from build123d import *

# Parameters (mm, degrees)
F1_DEPTH     = 25
F2_T1_DEPTH  = 30
F2_T3_DEPTH  = 30
F2_T5_DEPTH  = 30
F2_T7_DEPTH  = 30
F2_T9_DEPTH  = 30
F2_T11_DEPTH = 30
F2_T13_DEPTH = 30
F2_T15_DEPTH = 30
F2_T17_DEPTH = 30
F2_T19_DEPTH = 30
F2_T21_DEPTH = 30
F2_T23_DEPTH = 60.3553390593
F2_T25_DEPTH = 75


# Not quite as in the source:
# - a fillet or chamfer that OpenCascade refuses, or shapes differently, is made with other operations: its cross-section is extruded or revolved along the edge and cut away or added


with BuildPart() as f1:
    # F0 (on Top) → F1 (new body, symmetric)
    with BuildSketch(Plane.XY):
        Polygon((-96.1758106947, -16.0049479455), (-96.1758106947, -21.0049479455), (103.8241893053, -21.0049479455), (103.8241893053, -16.0049479455), (98.8241893053, -16.0049479455), (84.3241893053, -16.0049479455), (79.3241893053, -16.0049479455), (64.8241893053, -16.0049479455), (59.8241893053, -16.0049479455), (45.3241893053, -16.0049479455), (40.3241893053, -16.0049479455), (25.8241893053, -16.0049479455), (20.8241893053, -16.0049479455), (6.3241893053, -16.0049479455), (1.3241893053, -16.0049479455), (-13.1758106947, -16.0049479455), (-18.1758106947, -16.0049479455), (-32.6758106947, -16.0049479455), (-37.6758106947, -16.0049479455), (-52.1758106947, -16.0049479455), (-57.1758106947, -16.0049479455), (-71.6758106947, -16.0049479455), (-76.6758106947, -16.0049479455), (-91.1758106947, -16.0049479455), align=None)
        Polygon((-51.1758106947, 28.9950520545), (-96.1758106947, -16.0049479455), (-91.1758106947, -16.0049479455), (-46.1758106947, 28.9950520545), align=None)
        Polygon((98.8241893053, -16.0049479455), (103.8241893053, -16.0049479455), (148.8241893053, 28.9950520545), (143.8241893053, 28.9950520545), align=None)
        Polygon((-31.6758106947, 28.9950520545), (-76.6758106947, -16.0049479455), (-71.6758106947, -16.0049479455), (-26.6758106947, 28.9950520545), align=None)
        Polygon((79.3241893053, -16.0049479455), (84.3241893053, -16.0049479455), (129.3241893053, 28.9950520545), (124.3241893053, 28.9950520545), align=None)
        Polygon((-12.1758106947, 28.9950520545), (-57.1758106947, -16.0049479455), (-52.1758106947, -16.0049479455), (-7.1758106947, 28.9950520545), align=None)
        Polygon((59.8241893053, -16.0049479455), (64.8241893053, -16.0049479455), (109.8241893053, 28.9950520545), (104.8241893053, 28.9950520545), align=None)
        Polygon((7.3241893053, 28.9950520545), (-37.6758106947, -16.0049479455), (-32.6758106947, -16.0049479455), (12.3241893053, 28.9950520545), align=None)
        Polygon((40.3241893053, -16.0049479455), (45.3241893053, -16.0049479455), (90.3241893053, 28.9950520545), (85.3241893053, 28.9950520545), align=None)
        Polygon((26.8241893053, 28.9950520545), (-18.1758106947, -16.0049479455), (-13.1758106947, -16.0049479455), (31.8241893053, 28.9950520545), align=None)
        Polygon((20.8241893053, -16.0049479455), (25.8241893053, -16.0049479455), (70.8241893053, 28.9950520545), (65.8241893053, 28.9950520545), align=None)
        Polygon((46.3241893053, 28.9950520545), (1.3241893053, -16.0049479455), (6.3241893053, -16.0049479455), (51.3241893053, 28.9950520545), align=None)
    extrude(amount=F1_DEPTH, both=True)

    # F2: fillet of radius 5 on 25 edges, made by hand

    # F2_s2 → F2_t1 (cut)
    with BuildSketch(Plane.YZ.offset(-63.6758106947)):
        with BuildLine():
            ThreePointArc((28.9950520545, 20), (27.5305859605, 23.5355339059), (23.9950520545, 25))
            Line((23.9950520545, 25), (28.9950520545, 25))
            Line((28.9950520545, 25), (28.9950520545, 20))
        make_face()
        with BuildLine():
            ThreePointArc((28.9950520545, -20), (27.5305859605, -23.5355339059), (23.9950520545, -25))
            Line((23.9950520545, -25), (28.9950520545, -25))
            Line((28.9950520545, -25), (28.9950520545, -20))
        make_face()
    extrude(amount=F2_T1_DEPTH, mode=Mode.SUBTRACT)

    # F2_s4 → F2_t3 (cut)
    with BuildSketch(Plane.YZ.offset(-44.1758106947)):
        with BuildLine():
            ThreePointArc((28.9950520545, 20), (27.5305859605, 23.5355339059), (23.9950520545, 25))
            Line((23.9950520545, 25), (28.9950520545, 25))
            Line((28.9950520545, 25), (28.9950520545, 20))
        make_face()
        with BuildLine():
            ThreePointArc((28.9950520545, -20), (27.5305859605, -23.5355339059), (23.9950520545, -25))
            Line((23.9950520545, -25), (28.9950520545, -25))
            Line((28.9950520545, -25), (28.9950520545, -20))
        make_face()
    extrude(amount=F2_T3_DEPTH, mode=Mode.SUBTRACT)

    # F2_s6 → F2_t5 (cut)
    with BuildSketch(Plane.YZ.offset(-24.6758106947)):
        with BuildLine():
            ThreePointArc((28.9950520545, 20), (27.5305859604, 23.5355339059), (23.9950520545, 25))
            Line((23.9950520545, 25), (28.9950520545, 25))
            Line((28.9950520545, 25), (28.9950520545, 20))
        make_face()
        with BuildLine():
            ThreePointArc((28.9950520545, -20), (27.5305859604, -23.5355339059), (23.9950520545, -25))
            Line((23.9950520545, -25), (28.9950520545, -25))
            Line((28.9950520545, -25), (28.9950520545, -20))
        make_face()
    extrude(amount=F2_T5_DEPTH, mode=Mode.SUBTRACT)

    # F2_s8 → F2_t7 (cut)
    with BuildSketch(Plane.YZ.offset(-5.1758106947)):
        with BuildLine():
            ThreePointArc((28.9950520545, 20), (27.5305859604, 23.5355339059), (23.9950520545, 25))
            Line((23.9950520545, 25), (28.9950520545, 25))
            Line((28.9950520545, 25), (28.9950520545, 20))
        make_face()
        with BuildLine():
            ThreePointArc((28.9950520545, -20), (27.5305859604, -23.5355339059), (23.9950520545, -25))
            Line((23.9950520545, -25), (28.9950520545, -25))
            Line((28.9950520545, -25), (28.9950520545, -20))
        make_face()
    extrude(amount=F2_T7_DEPTH, mode=Mode.SUBTRACT)

    # F2_s10 → F2_t9 (cut)
    with BuildSketch(Plane.YZ.offset(14.3241893053)):
        with BuildLine():
            ThreePointArc((28.9950520545, 20), (27.5305859605, 23.5355339059), (23.9950520545, 25))
            Line((23.9950520545, 25), (28.9950520545, 25))
            Line((28.9950520545, 25), (28.9950520545, 20))
        make_face()
        with BuildLine():
            ThreePointArc((28.9950520545, -20), (27.5305859605, -23.5355339059), (23.9950520545, -25))
            Line((23.9950520545, -25), (28.9950520545, -25))
            Line((28.9950520545, -25), (28.9950520545, -20))
        make_face()
    extrude(amount=F2_T9_DEPTH, mode=Mode.SUBTRACT)

    # F2_s12 → F2_t11 (cut)
    with BuildSketch(Plane.YZ.offset(33.8241893053)):
        with BuildLine():
            ThreePointArc((28.9950520545, 20), (27.5305859605, 23.5355339059), (23.9950520545, 25))
            Line((23.9950520545, 25), (28.9950520545, 25))
            Line((28.9950520545, 25), (28.9950520545, 20))
        make_face()
        with BuildLine():
            ThreePointArc((28.9950520545, -20), (27.5305859605, -23.5355339059), (23.9950520545, -25))
            Line((23.9950520545, -25), (28.9950520545, -25))
            Line((28.9950520545, -25), (28.9950520545, -20))
        make_face()
    extrude(amount=F2_T11_DEPTH, mode=Mode.SUBTRACT)

    # F2_s14 → F2_t13 (cut)
    with BuildSketch(Plane.YZ.offset(53.3241893053)):
        with BuildLine():
            ThreePointArc((28.9950520545, 20), (27.5305859605, 23.5355339059), (23.9950520545, 25))
            Line((23.9950520545, 25), (28.9950520545, 25))
            Line((28.9950520545, 25), (28.9950520545, 20))
        make_face()
        with BuildLine():
            ThreePointArc((28.9950520545, -20), (27.5305859605, -23.5355339059), (23.9950520545, -25))
            Line((23.9950520545, -25), (28.9950520545, -25))
            Line((28.9950520545, -25), (28.9950520545, -20))
        make_face()
    extrude(amount=F2_T13_DEPTH, mode=Mode.SUBTRACT)

    # F2_s16 → F2_t15 (cut)
    with BuildSketch(Plane.YZ.offset(72.8241893053)):
        with BuildLine():
            ThreePointArc((28.9950520545, 20), (27.5305859605, 23.5355339059), (23.9950520545, 25))
            Line((23.9950520545, 25), (28.9950520545, 25))
            Line((28.9950520545, 25), (28.9950520545, 20))
        make_face()
        with BuildLine():
            ThreePointArc((28.9950520545, -20), (27.5305859605, -23.5355339059), (23.9950520545, -25))
            Line((23.9950520545, -25), (28.9950520545, -25))
            Line((28.9950520545, -25), (28.9950520545, -20))
        make_face()
    extrude(amount=F2_T15_DEPTH, mode=Mode.SUBTRACT)

    # F2_s18 → F2_t17 (cut)
    with BuildSketch(Plane.YZ.offset(92.3241893053)):
        with BuildLine():
            ThreePointArc((28.9950520545, 20), (27.5305859605, 23.5355339059), (23.9950520545, 25))
            Line((23.9950520545, 25), (28.9950520545, 25))
            Line((28.9950520545, 25), (28.9950520545, 20))
        make_face()
        with BuildLine():
            ThreePointArc((28.9950520545, -20), (27.5305859605, -23.5355339059), (23.9950520545, -25))
            Line((23.9950520545, -25), (28.9950520545, -25))
            Line((28.9950520545, -25), (28.9950520545, -20))
        make_face()
    extrude(amount=F2_T17_DEPTH, mode=Mode.SUBTRACT)

    # F2_s20 → F2_t19 (cut)
    with BuildSketch(Plane.YZ.offset(111.8241893053)):
        with BuildLine():
            ThreePointArc((28.9950520545, 20), (27.5305859605, 23.5355339059), (23.9950520545, 25))
            Line((23.9950520545, 25), (28.9950520545, 25))
            Line((28.9950520545, 25), (28.9950520545, 20))
        make_face()
        with BuildLine():
            ThreePointArc((28.9950520545, -20), (27.5305859605, -23.5355339059), (23.9950520545, -25))
            Line((23.9950520545, -25), (28.9950520545, -25))
            Line((28.9950520545, -25), (28.9950520545, -20))
        make_face()
    extrude(amount=F2_T19_DEPTH, mode=Mode.SUBTRACT)

    # F2_s22 → F2_t21 (cut)
    with BuildSketch(Plane.YZ.offset(131.3241893053)):
        with BuildLine():
            ThreePointArc((28.9950520545, 20), (27.5305859605, 23.5355339059), (23.9950520545, 25))
            Line((23.9950520545, 25), (28.9950520545, 25))
            Line((28.9950520545, 25), (28.9950520545, 20))
        make_face()
        with BuildLine():
            ThreePointArc((28.9950520545, -20), (27.5305859605, -23.5355339059), (23.9950520545, -25))
            Line((23.9950520545, -25), (28.9950520545, -25))
            Line((28.9950520545, -25), (28.9950520545, -20))
        make_face()
    extrude(amount=F2_T21_DEPTH, mode=Mode.SUBTRACT)

    # F2_s24 → F2_t23 (cut)
    with BuildSketch(Plane.XY.offset(-30.1776695297)):
        with BuildLine():
            ThreePointArc((-96.1758106947, -18.0760157573), (-95.7952083573, -16.1625985955), (-94.7113446006, -14.5404818514))
            Line((-94.7113446006, -14.5404818514), (-96.1758106947, -16.0049479455))
            Line((-96.1758106947, -16.0049479455), (-96.1758106947, -18.0760157573))
        make_face()
    extrude(amount=F2_T23_DEPTH, mode=Mode.SUBTRACT)

    # F2_s26 → F2_t25 (cut)
    with BuildSketch(Plane.XY.offset(-37.5)):
        with BuildLine():
            ThreePointArc((-96.1758106947, -16.0049479455), (-94.7113446006, -19.5404818514), (-91.1758106947, -21.0049479455))
            Line((-91.1758106947, -21.0049479455), (-96.1758106947, -21.0049479455))
            Line((-96.1758106947, -21.0049479455), (-96.1758106947, -16.0049479455))
        make_face()
        with BuildLine():
            ThreePointArc((103.8241893053, -16.0049479455), (102.3597232112, -19.5404818514), (98.8241893053, -21.0049479455))
            Line((98.8241893053, -21.0049479455), (103.8241893053, -21.0049479455))
            Line((103.8241893053, -21.0049479455), (103.8241893053, -16.0049479455))
        make_face()
    extrude(amount=F2_T25_DEPTH, mode=Mode.SUBTRACT)


solid = f1.part
Here's how the part is built. I have some questions about the finished solid (model axes, mm). A direction names the side the tool comes from. Give positions to 0.01 mm unless a question says otherwise; leave off trailing zeros. Order: outer loops, then holes, each group sorted by start corner. A loop starts at its lowest first (then second) coordinate and runs counter-clockwise, first axis right, second up. Notation, with made-up numbers: (2, -3.5) -> (11, -3.5) arc R15 cw to (11, 25.5) -> close; hole circle Ø1 at (77, 65). An arc over 180 degrees is marked (long way). Use a Markdown table: item, result. Add a question column.
Item 1: I need wall thicknesses on line 1 (Y direction, x = -19, z = 15); line 2 (Y direction, x = 96.5, z = -8.5); line 3 (Y direction, x = 9, z = -22). Which ranges of each line are inside material? Lowest first, please.
Item 2: Imagine slicing it at A-A on x = 57. Please give me the cut outline in (y, z).
Item 3: Will these pins go through, and if not, where does the flat tip stop? pin 1 (4 mm diameter, centred on x = -48.5, y = -14.5, fed in from +Z); pin 2 (4.5 mm diameter, centred on x = 94.5, z = -5, fed in from +Y); pin 3 (1 mm diameter, centred on x = -21.5, z = -3.5, fed in from +Y); pin 4 (11.5 mm diameter, centred on x = -83.5, z = -11, fed in from +Y).
Item 4: For faces 5 (the face through (-30.635, 27.569, 23.496)), 6 (the face through (48.01, 6.18, 0.35)), which set-ups out of +Z, -Z, +X, -X, +Y, -Y let a thin tool reach every point of the face, with its end or its side?
Item 5: Imagine slicing it at B-B on y = -7. Give the number of separate pieces and of enclosed holes in the cut face, plus the area to 3 significant figures.
Item 6: If we mould it in two halves opening along Y, with no side actions, what happens to faces 1 (the face through (-94.36, -19.86, -0.35)), 2 (the face through (-68.99, 6.18, 0.35)), 3 (the face through (-14.86, 6.81, 0.35)), 4 (the face through (105.865, 27.569, -23.496))? For each: pulls with the +Y half, pulls with the -Y half, needs draft (parallel to the pull), parting line crosses it, or undercut.
Data:
| question | item | result |
|---|---|---|
| 1 | line 1 | y = -21 to -16, -2.33 to 2.67, 17.17 to 22.17 |
| 1 | line 2 | y = -21 to -16, -3.83 to 1.17, 15.67 to 20.67 |
| 1 | line 3 | y = -21 to -16, -13.33 to -8.33, 6.17 to 11.17, 25.67 to 28.58 |
| 2 | outline | (-21, -25) -> (-16, -25) -> (-16, 25) -> (-21, 25) -> close; (-4.33, -25) -> (0.67, -25) -> (0.67, 25) -> (-4.33, 25) -> close; (15.17, -25) -> (20.17, -25) -> (20.17, 25) -> (15.17, 25) -> close |
| 3 | pin 1 | stops at z = 25 |
| 3 | pin 2 | stops at y = 20.92 |
| 3 | pin 3 | stops at y = 20.17 |
| 3 | pin 4 | stops at y = 2.42 |
| 4 | face 5 | +Z, +X, -X, +Y |
| 4 | face 6 | +Z, -Z |
| 5 | separate pieces | 11 |
| 5 | enclosed holes | 0 |
| 5 | area | 2,750 mm² |
| 6 | face 1 | pulls with the -Y half |
| 6 | face 2 | undercut |
| 6 | face 3 | undercut |
| 6 | face 4 | pulls with the +Y half |
